CAD build for the part. Positions are in the model's coordinates, mm. A direction names the side the tool comes from. Coordinates: 2 decimals unless noted, no trailing zeros. Write each loop counter-clockwise with the first axis right and the second up, starting at its lowest first coordinate (ties: lowest second). Pieces come first, ordered by that corner, then holes. Notation, with made-up numbers: M 50.5,85 L 82.5,85 A28 cw 82.5,104 Z; hole C 76,16.25 d7. An arc over 180 degrees is marked long. Put each result on its own line as item: value. Start each with the question number.
Autodesk Inventor part; units mm, degrees
ref_plane "YZ Plane" through (0, 0, 0) normal (1, 0, 0) x (0, 1, 0)
ref_plane "XZ Plane" through (0, 0, 0) normal (0, 1, 0) x (-1, 0, 0)
ref_plane "XY Plane" through (0, 0, 0) normal (0, 0, 1) x (1, 0, 0)
sketch "Sketch1" plane through (0, 0, 0) normal (0, 0, 1) x (1, 0, 0)
  circle A0 centre (0, 0) radius 2.5
  line L0 (-1.5, 2) -> (1.5, 2)
  dimension "d0" = 5
sketch "Sketch1 outline for Extrusion1" plane through (0, 0, 0) normal (0, 0, 1) x (1, 0, 0)
  line L0 (1.5, 2) -> (-1.5, 2)
  arc A0 (-1.5, 2) -> (1.5, 2) centre (0, 0) ccw
extrude "Extrusion1" add sketch "Sketch1 outline for Extrusion1" along normal blind 24
sketch "Sketch2" plane through (0, 0, 0) normal (0, 0, -1) x (-1, 0, 0)
  line L0 (-1.5, 2) -> (1.5, 2)
  arc A0 (-1.5, 2) -> (1.5, 2) centre (0, 0) ccw
  arc A1 (1.5, 2) -> (-1.5, 2) centre (0, 0) ccw
  dimension "d3" = 2.5
sketch "Sketch2 outline for Extrusion2" plane through (0, 0, 0) normal (0, 0, -1) x (-1, 0, 0)
  line L0 (-1.5, 2) -> (1.5, 2)
  arc A0 (1.5, 2) -> (-1.5, 2) centre (0, 0) ccw
extrude "Extrusion2" add sketch "Sketch2 outline for Extrusion2" against normal blind 6
chamfer "Chamfer1" distance 0.5 angle 45 1 edges at (0, -2.5, 24)
properties part number "Stepper Motor Shaft"
(1) Drill centre lines: line 1 (X direction, y = 1.5, z = 11); line 2 (Z direction, x = -0.55, y = 2.25); line 3 (X direction, y = -2, z = 8.25). Where is each one in solid material? Low to high. Write a range as [from, to].
(2) Slice it at A-A, the plane z = 4.5. Write the cut outline in (x, y).
(3) Drop flat-ended pins along their axis: pin 1 (2 mm diameter, centred on x = -1, z = 21, fed in from +Y); pin 2 (2 mm diameter, centred on x = 0.5, y = 1.5, fed in from -Z); pin 3 (1 mm diameter, centred on y = 1.5, z = 18, fed in from +X). Give the stop position or say it passes through.
(4) Which spindle directions (+Z, -Z, +X, -X, +Y, -Y) get a long thin tool onto all of the face, cutting with end or side? Do faces 1 (the face through (0, 2, 15)), 2 (the face through (0, -2.5, 11.6)). Say none if no direction does.
(5) Slice it at B-B, the plane z = 11.5. Write the cut outline in (x, y).
Result set:
1. line 1: x = [-2, 2]
1. line 2: z = [0, 6]
1. line 3: x = [-1.5, 1.5]
2. outline: C 0,0 d5
3. pin 1: stops at y = 2
3. pin 2: stops at z = 0
3. pin 3: stops at x = 2.29
4. face 1: +Z, +X, -X, +Y
4. face 2: +Z, -Z
5. outline: M -1.5,2 A2.5 ccw long 1.5,2 Z
